```python
from build123d import *

# Parameters (mm, degrees)
F1_ANGLE = 180


with BuildPart() as f1:
    # F0 (on Front) → F1 (revolve, symmetric)
    with BuildSketch(Plane.XZ) as f1_sk:
        with BuildLine():
            ThreePointArc((-15, 93.658174), (-32.67767, 86.335844), (-40, 68.658174))
            Line((-40, 68.658174), (-40, -56.341826))
            ThreePointArc((-40, -56.341826), (-32.67767, -74.019496), (-15, -81.341826))
            Line((-15, -81.341826), (55, -81.341826))
            Line((55, -81.341826), (55, -61.341826))
            Line((55, -61.341826), (-20, -61.341826))
            Line((-20, -61.341826), (-20, 73.658174))
            Line((-20, 73.658174), (-5, 73.658174))
            ThreePointArc((-5, 73.658174), (12.67767, 80.980504), (20, 98.658174))
            Line((20, 98.658174), (20, 128.658174))
            ThreePointArc((20, 128.658174), (30, 138.658174), (20, 148.658174))
            Line((20, 148.658174), (0, 148.658174))
            Line((0, 148.658174), (0, 93.658174))
            Line((0, 93.658174), (-15, 93.658174))
        make_face()
    revolve(axis=Axis((55, 0, -71.341826), (0, 0, 1)), revolution_arc=F1_ANGLE / 2)
    revolve(f1_sk.sketch, axis=Axis((55, 0, -71.341826), (0, 0, -1)), revolution_arc=F1_ANGLE / 2)


solid = f1.part
```
Part model, mm, in its own coordinate system. A direction names the side the tool comes from. Round coordinates to 2 decimals unless told otherwise and drop trailing zeros. Loops run counter-clockwise (first coordinate to the right, second up) from the corner with the lowest first, then second, coordinate; pieces in that order, holes last. Notation, with made-up numbers: (-39, 32) -> (0, 32) arc R12 cw to (0, 45) -> close; hole circle Ø1 at (-29.75, 59). An arc over 180 degrees is marked (long way). Use one line per item in the form item = value. Start each with the question number.
Item 1: Two-plate mould, pull along Z, no slides. Class faces 1 (the cylindrical face through (20.01, -0.77, 113.87)), 2 (the cylindrical face through (0.013, -1.209, 120.773)), 3 (the cylindrical face through (-19.98, -1.65, 7.1)), 4 (the flat face through (28, 1, -81.342)): released by +Z, released by -Z, zero draft, split by the parting line, or undercut.
Item 2: Drop flat-ended pins along their axis: pin 1 Ø21 at (x, y) = (3.5, -28) entering from +Z; pin 2 Ø5 at (x, z) = (27.5, 15.5) entering from -Y; pin 3 Ø10 at (x, z) = (-21, 44) entering from +Y; pin 4 Ø8 at (x, y) = (-11, -46.5) entering from -Z. Give the stop position or say it passes through.
Item 3: Drill centre lines: line 1 along Z through (x, y) = (-7, 1.5); line 2 along Z through (x, y) = (-16, 8.5); line 3 along Y through (x, z) = (-12.5, 56). Where is each one in solid material? Low to high.
Item 4: Band-saw the part on B-B (z = 118). List the corners of the cut face in (x, y).
Item 5: Tool access for faces 5 (the cylindrical face through (-39.977, -2.089, 5.283)), 6 (the flat face through (-1, 0, 93.658)), 7 (the flat face through (-5, 11, 73.658)): list every direction of +Z, -Z, +X, -X, +Y, -Y with a clear straight run to the whole face (end or side of a thin tool).
Item 6: Band-saw the part on C-C (z = -48.5). List the corners of the cut face in (x, y), plus the area to 3 significant figures.
Item 7: Band-saw the part on A-A (y = 0). List the corners of the cut face in (x, z).
Data:
q1.face_1 = undercut
q1.face_2 = zero draft
q1.face_3 = undercut
q1.face_4 = released by -Z
q2.pin_1 = 148.66
q2.pin_2 = -91.65
q2.pin_3 = 63.12
q2.pin_4 = -80.42
q3.line_1 = -81.34 to -61.34, 73.66 to 93.66
q3.line_2 = -81.3 to -61.34, 73.66 to 93.61
q3.line_3 = -66.85 to -32.69, 32.69 to 66.85
q4.outline = (55, -55) -> (55, -35) arc R35 cw to (55, 35) -> (55, 55) arc R55 ccw to start
q5.face_5 = +Z, -Z, -X
q5.face_6 = +Z, -X
q5.face_7 = +X
q6.outline = (55, -95) -> (55, -75) arc R75 cw to (55, 75) -> (55, 95) arc R95 ccw to start
q6.area = 5,340 mm^2
q7.outline = (-40, -56.34) arc R25 ccw to (-15, -81.34) -> (55, -81.34) -> (55, -61.34) -> (-20, -61.34) -> (-20, 73.66) -> (-5, 73.66) arc R25 ccw to (20, 98.66) -> (20, 128.66) arc R10 ccw to (20, 148.66) -> (0, 148.66) -> (0, 93.66) -> (-15, 93.66) arc R25 ccw to (-40, 68.66) -> close
